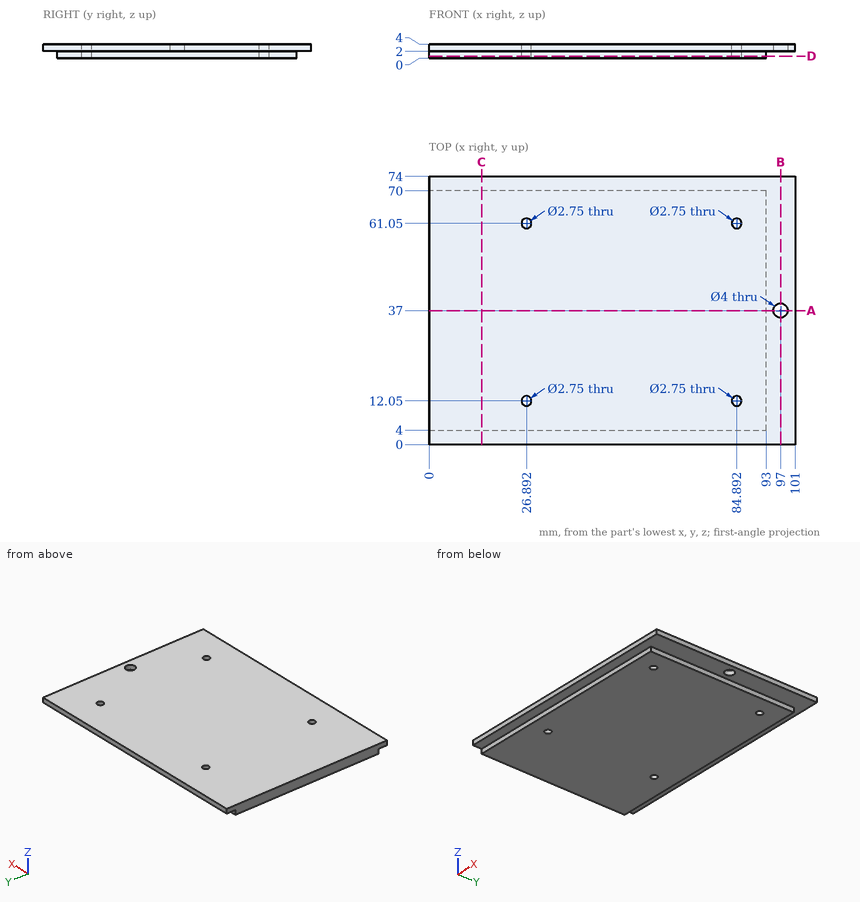
Geometry check sheet. Reference: drawing and pictorial views, mm from the part's lowest x, y, z. Coordinates: 2 decimals unless noted, no trailing zeros. Loops run counter-clockwise (first coordinate to the right, second up) from the corner with the lowest first, then second, coordinate; pieces in that order, holes last. Notation, with made-up numbers: M 12,54 L 33,54 A24 cw 33,79 Z; hole C 6,5.25 d7. An arc over 180 degrees is marked long. One line per item, written item: value.
1. Section check B-B on x = 97. Record the cut outline in (y, z), plus the area to 3 significant figures.
Answers follow:
outline: M 0,2 L 35,2 L 35,4 L 0,4 Z; M 39,2 L 74,2 L 74,4 L 39,4 Z
area: 140 mm^2
2. Gauge pin test, flat ends, axial feed: P1, Ø0.6, axis at x = 66, z = 1, coming from the -Y side; P2, Ø1, axis at x = 51.5, z = 1, coming from the +Y side; P3, Ø0.6, axis at y = 31, z = 1.5, coming from the +X side. Record the tip position at first contact, or that the pin passes through.
Answers follow:
P1: y = 4
P2: y = 70
P3: x = 93
3. Section check D-D on z = 0.65. Give the number of separate pieces and of enclosed holes in the cut face, plus the area to 3 significant figures.
Answers follow:
separate pieces: 1
enclosed holes: 4
area: 6,110 mm^2
4. Section check C-C on x = 14.5. Record the cut outline in (y, z).
Answers follow:
outline: M 0,2 L 4,2 L 4,0 L 70,0 L 70,2 L 74,2 L 74,4 L 0,4 Z
5. Material ranges on line 1 along Y through (x, z) = (27, 1.95); line 2 along Y through (x, z) = (97, 2.6); line 3 along X through (y, z) = (62, 0.2) (1 decimal), recorded low to high. Write a range as from..to.
Answers follow:
line 1: 4..10.68, 13.42..59.68, 62.42..70
line 2: 0..35, 39..74
line 3: 0..25.9, 27.9..83.9, 85.9..93
6. Section check A-A on y = 37. Record the cut outline in (x, z), plus the area to 3 significant figures.
Answers follow:
outline: M 0,0 L 93,0 L 93,2 L 95,2 L 95,4 L 0,4 Z; M 99,2 L 101,2 L 101,4 L 99,4 Z
area: 380 mm^2
